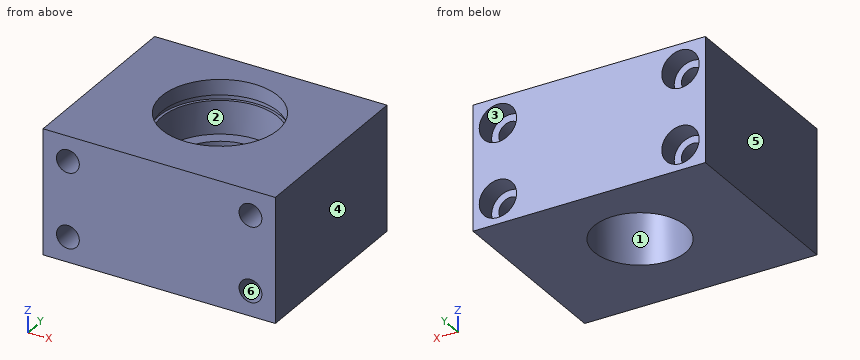
```python
from build123d import *

# Parameters (mm, degrees)
SZKIC1_W                                             = 56
SZKIC1_H                                             = 30
DODANIE_WYCI_GNI_CIE1_DEPTH                          = 45
SZKIC3_R                                             = 11
WYTNIJ_WYCI_GNI_CIE2_DEPTH                           = 61.901559914
SZKIC4_R                                             = 14
WYTNIJ_WYCI_GNI_CIE3_DEPTH                           = 13
POG_BIENIE_WALCOWE_POD_M5_WKR_T_DO_CZ_CI_D           = 5.5
POG_BIENIE_WALCOWE_POD_M5_WKR_T_DO_CZ_CI_CBORE_D     = 9
POG_BIENIE_WALCOWE_POD_M5_WKR_T_DO_CZ_CI_CBORE_DEPTH = 5
SZKIC5_W                                             = 1.3
SZKIC5_H                                             = 0.7


with BuildPart() as part:
    # Szkic1 → Dodanie-wyciągnięcie1 (new body)
    with BuildSketch(Plane(origin=(0, 0, 0), x_dir=(1, 0, 0), z_dir=(0, 1, 0))):
        Rectangle(SZKIC1_W, SZKIC1_H)
    extrude(amount=DODANIE_WYCI_GNI_CIE1_DEPTH)

    # Szkic3 → Wytnij-wyciągnięcie2 (cut, through all)
    with BuildSketch(Plane.XY.offset(15)):
        with Locations((0, 24.5)):
            Circle(SZKIC3_R)
    extrude(amount=-WYTNIJ_WYCI_GNI_CIE2_DEPTH, mode=Mode.SUBTRACT)

    # Szkic4 → Wytnij-wyciągnięcie3 (cut)
    with BuildSketch(Plane.XY.offset(15)):
        with Locations((0, 24.5)):
            Circle(SZKIC4_R)
    extrude(amount=-WYTNIJ_WYCI_GNI_CIE3_DEPTH, mode=Mode.SUBTRACT)

    # Pogłębienie walcowe pod M5 Wkręt do części metalowych z łbem sześciokątnym1 (through all)
    with Locations(Plane(origin=(0, 45, 0), x_dir=(1, 0, 0), z_dir=(0, 1, 0))):
        with Locations((22, 9), (22, -9), (-22, -9), (-22, 9)):
            CounterBoreHole(POG_BIENIE_WALCOWE_POD_M5_WKR_T_DO_CZ_CI_D / 2, POG_BIENIE_WALCOWE_POD_M5_WKR_T_DO_CZ_CI_CBORE_D / 2, POG_BIENIE_WALCOWE_POD_M5_WKR_T_DO_CZ_CI_CBORE_DEPTH)

    # Szkic5 → Wycięcie-obrót1 (revolve, cut)
    with BuildSketch(Plane(origin=(0, 0, 0), x_dir=(0, 0, -1), z_dir=(1, 0, 0)), mode=Mode.PRIVATE) as wyci_cie_obr_t1_sk:
        with Locations((-10.65, 10.15)):
            Rectangle(SZKIC5_W, SZKIC5_H)
    revolve(wyci_cie_obr_t1_sk.sketch.rotate(Axis((0, 24.5, 9.294649117), (0, 0, 1)), 90), axis=Axis((0, 24.5, 9.294649117), (0, 0, 1)), mode=Mode.SUBTRACT)


solid = part.part
```
For this review, take the finished solid that the model builds, in its own axes (mm). Face numbers are marked on the shaded views. A direction names the side the tool comes from. Coordinates: 2 decimals unless noted, no trailing zeros. Loops run counter-clockwise (first coordinate to the right, second up) from the corner with the lowest first, then second, coordinate; pieces in that order, holes last. Notation, with made-up numbers: (33.5, -10) -> (60.5, -10) arc R19 cw to (60.5, 14) -> close; hole circle Ø8 at (-2.75, 45). An arc over 180 degrees is marked (long way). Return JSON: item names as keys, results as strings. Group by question number.
(1) Consider section C-C, the plane x = 22. Give the boundary of the cut face in (y, z).
(2) Consider section A-A, the plane y = 24.5. Give the boundary of the cut face in (x, z), plus the area to 3 significant figures.
(3) Consider section D-D, the plane x = 0. Give the boundary of the cut face in (y, z).
(4) To check wall thickness, follow L1, parallel to Z at x = -22, y = 26; L2, parallel to X at y = 9, z = -8.75; L3, parallel to Y at x = 0, z = 4. State the ranges of each line that lie inside material, in increasing order.
(5) For pin 1 Ø7 at (x, z) = (22, 9) entering from +Y; pin 2 Ø17.5 at (x, y) = (0, 24.5) entering from +Z; pin 3 Ø23.5 at (x, y) = (0, 24.5) entering from +Z, all flat-tipped, find the tip position at first contact; note any pin that passes through.
(6) Consider section B-B, the plane z = 9. Give the boundary of the cut face in (x, y).
(7) Mouldability with a two-part tool opening along X and no side actions: class the marked faces 4, 5 and 6 as pulls with the +X half, pulls with the -X half, needs draft (parallel to the pull), parting line crosses it, or undercut.
(8) Tool access review of the marked faces 1, 2 and 3: name each direction out of +Z, -Z, +X, -X, +Y, -Y from which nothing blocks a thin tool from reaching the whole face with its end or side.
Results below:
{
 "1": {"outline": "(0, -15) -> (45, -15) -> (45, -13.5) -> (40, -13.5) -> (40, -11.75) -> (0, -11.75) -> close; (0, -6.25) -> (40, -6.25) -> (40, -4.5) -> (45, -4.5) -> (45, 4.5) -> (40, 4.5) -> (40, 6.25) -> (0, 6.25) -> close; (0, 11.75) -> (40, 11.75) -> (40, 13.5) -> (45, 13.5) -> (45, 15) -> (0, 15) -> close"},
 "2": {"outline": "(-28, -15) -> (-11, -15) -> (-11, 2) -> (-14, 2) -> (-14, 10) -> (-14.7, 10) -> (-14.7, 11.3) -> (-14, 11.3) -> (-14, 15) -> (-28, 15) -> close; (11, -15) -> (28, -15) -> (28, 15) -> (14, 15) -> (14, 11.3) -> (14.7, 11.3) -> (14.7, 10) -> (14, 10) -> (14, 2) -> (11, 2) -> close; hole circle Ø5.5 at (-22, -9); hole circle Ø5.5 at (-22, 9); hole circle Ø5.5 at (22, -9); hole circle Ø5.5 at (22, 9)", "area": "845 mm2"},
 "3": {"outline": "(0, -15) -> (13.5, -15) -> (13.5, 2) -> (10.5, 2) -> (10.5, 10) -> (9.8, 10) -> (9.8, 11.3) -> (10.5, 11.3) -> (10.5, 15) -> (0, 15) -> close; (35.5, -15) -> (45, -15) -> (45, 15) -> (38.5, 15) -> (38.5, 11.3) -> (39.2, 11.3) -> (39.2, 10) -> (38.5, 10) -> (38.5, 2) -> (35.5, 2) -> close"},
 "4": {"L1": "z = -15 to -11.75, -6.25 to 6.25, 11.75 to 15", "L2": "x = -28 to -24.74, -19.26 to 19.26, 24.74 to 28", "L3": "y = 0 to 10.5, 38.5 to 45"},
 "5": {"pin 1": "stops at y = 40", "pin 2": "passes through", "pin 3": "stops at z = 2"},
 "6": {"outline": "(-28, 0) -> (-24.75, 0) -> (-24.75, 40) -> (-26.5, 40) -> (-26.5, 45) -> (-28, 45) -> close; (-19.25, 0) -> (19.25, 0) -> (19.25, 40) -> (17.5, 40) -> (17.5, 45) -> (-17.5, 45) -> (-17.5, 40) -> (-19.25, 40) -> close; (24.75, 0) -> (28, 0) -> (28, 45) -> (26.5, 45) -> (26.5, 40) -> (24.75, 40) -> close; hole circle Ø28 at (0, 24.5)"},
 "7": {"face 4": "pulls with the +X half", "face 5": "pulls with the -X half", "face 6": "undercut"},
 "8": {"face 1": "+Z, -Z", "face 2": "+Z", "face 3": "+Y"}
}
